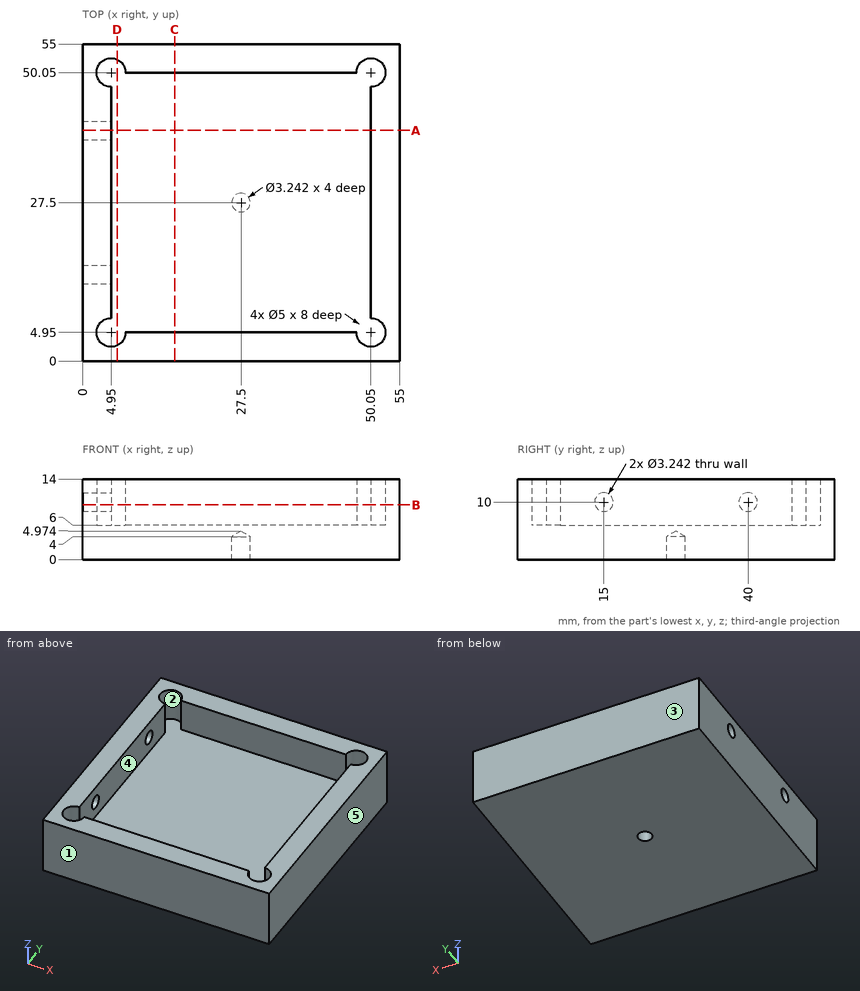
Design review of the part shown in the three views and the two pictorial views. Dimensions are in mm from the part's minimum x, y and z. A direction names the side the tool comes from. Round coordinates to 2 decimals unless told otherwise and drop trailing zeros. Write each loop counter-clockwise with the first axis right and the second up, starting at its lowest first coordinate (ties: lowest second). Pieces come first, ordered by that corner, then holes. Notation, with made-up numbers: (31.25, -19) -> (62.25, -19) arc R18 ccw to (62.25, 16) -> close; hole circle Ø10 at (15.5, -4). An arc over 180 degrees is marked (long way). Answer as a JSON object with one key per item and string values.
1. To check wall thickness, follow line 1 along Y through (x, z) = (13, 6.25); line 2 along Y through (x, z) = (27.5, 1). State the ranges of each line that lie inside material, in increasing order.
Results found:
{"line 1": "y = 0 to 4.95, 50.05 to 55", "line 2": "y = 0 to 25.88, 29.12 to 55"}
2. We need section B-B on z = 9.5. State the section outline as (x, y) points, and give its area (3 significant figures).
Results found:
{"outline": "(0, 0) -> (55, 0) -> (55, 55) -> (0, 55) -> (0, 41.54) -> (4.95, 41.54) -> (4.95, 47.55) arc R2.5 cw (long way) to (7.45, 50.05) -> (47.55, 50.05) arc R2.5 cw (long way) to (50.05, 47.55) -> (50.05, 7.45) arc R2.5 cw (long way) to (47.55, 4.95) -> (7.45, 4.95) arc R2.5 cw (long way) to (4.95, 7.45) -> (4.95, 13.46) -> (0, 13.46) -> close; (0, 16.54) -> (4.95, 16.54) -> (4.95, 38.46) -> (0, 38.46) -> close", "area": "902 mm^2"}
3. Clearance check with flat-ended pins moving along their axes: pin 1 (3 mm diameter, centred on x = 27.5, y = 27.5, fed in from -Z); pin 2 (4 mm diameter, centred on x = 18.5, y = 33.5, fed in from +Z). State where each tip first meets the part, or that it passes through.
Results found:
{"pin 1": "stops at z = 4.07", "pin 2": "stops at z = 6"}
4. We need section A-A on y = 40. State the section outline as (x, z) points.
Results found:
{"outline": "(0, 0) -> (55, 0) -> (55, 14) -> (50.05, 14) -> (50.05, 6) -> (4.95, 6) -> (4.95, 8.38) -> (0, 8.38) -> close; (0, 11.62) -> (4.95, 11.62) -> (4.95, 14) -> (0, 14) -> close"}
5. The part is to be moulded in two halves that separate along X. For the marked faces 3, 4 and 5, say which applies: pulls with the +X half, pulls with the -X half, needs draft (parallel to the pull), parting line crosses it, or undercut.
Results found:
{"face 3": "needs draft", "face 4": "undercut", "face 5": "pulls with the +X half"}
6. We need section C-C on x = 16. State the section outline as (y, z) points.
Results found:
{"outline": "(0, 0) -> (55, 0) -> (55, 14) -> (50.05, 14) -> (50.05, 6) -> (4.95, 6) -> (4.95, 14) -> (0, 14) -> close"}
7. Machinability: for the marked faces 1 and 2, which of the approach directions +Z, -Z, +X, -X, +Y, -Y give a long, thin tool a straight path to every point of the face, cutting with its end or side? Answer none if there is none.
Results found:
{"face 1": "+Z, -Z, +X, -X, -Y", "face 2": "+Z"}
8. We need section D-D on x = 6. State the section outline as (y, z) points, and give its area (3 significant figures).
Results found:
{"outline": "(0, 0) -> (55, 0) -> (55, 14) -> (52.32, 14) -> (52.32, 6) -> (2.68, 6) -> (2.68, 14) -> (0, 14) -> close", "area": "373 mm^2"}
